Geometry check sheet. Reference: the model listing, model coordinates, mm. Round coordinates to 2 decimals unless told otherwise and drop trailing zeros. Write each loop counter-clockwise with the first axis right and the second up, starting at its lowest first coordinate (ties: lowest second). Pieces come first, ordered by that corner, then holes. Notation, with made-up numbers: (16, 57.5) - (43, 57.5) arc R14 ccw to (43, 77.5) - close; hole circle Ø8 at (60, -16.5). An arc over 180 degrees is marked (long way). Return JSON: item names as keys, results as strings.
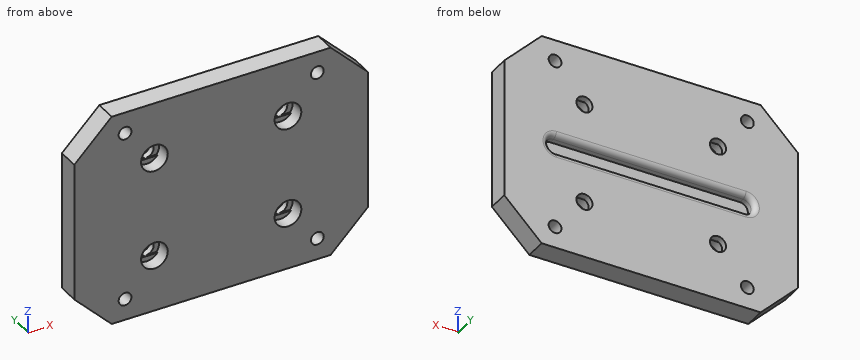
```python
from build123d import *

# Parameters (mm, degrees)
SKETCH2_W           = 55
SKETCH2_H           = 40
SKETCH2_R           = 1.2
BOSS_EXTRUDE1_DEPTH = 4
CHAMFER1_SIZE       = 7
SKETCH3_R           = 1.5
CUT_EXTRUDE1_DEPTH  = 35.062442661
FILLET1_R           = 1
CUT_EXTRUDE2_START  = 0.5
SKETCH4_R           = 2.5
CUT_EXTRUDE2_DEPTH  = 35.562442661
CUT_EXTRUDE6_START  = 0.3
CUT_EXTRUDE6_DEPTH  = 0.3


with BuildPart() as part:
    # Sketch2 → Boss-Extrude1 (new body)
    with BuildSketch(Plane(origin=(0, 0, 0), x_dir=(1, 0, 0), z_dir=(0, 1, 0))):
        Rectangle(SKETCH2_W, SKETCH2_H)
        with Locations(Location((-18, -16, 0), (0, 0, 270))):
            Circle(SKETCH2_R, mode=Mode.SUBTRACT)
        with Locations(Location((18, -16, 0), (0, 0, 270))):
            Circle(SKETCH2_R, mode=Mode.SUBTRACT)
        with Locations(Location((-18, 16, 0), (0, 0, 270))):
            Circle(SKETCH2_R, mode=Mode.SUBTRACT)
        with Locations(Location((18, 16, 0), (0, 0, 270))):
            Circle(SKETCH2_R, mode=Mode.SUBTRACT)
    extrude(amount=-BOSS_EXTRUDE1_DEPTH)

    # Chamfer1
    chamfer1_edges = [part.edges().sort_by_distance(p)[0] for p in [
        (27.5, -2, 20),
        (-27.5, -2, 20),
        (-27.5, -2, -20),
        (27.5, -2, -20),
    ]]
    chamfer(chamfer1_edges, length=CHAMFER1_SIZE)

    # Sketch3 → Cut-Extrude1 (cut, through all)
    with BuildSketch(Plane(origin=(0, -2, 0), x_dir=(1, 0, 0), z_dir=(0, 1, 0))):
        with Locations(Location((12.5, 9.4, 0), (0, 0, 270))):
            Circle(SKETCH3_R)
        with Locations(Location((-12.5, 9.4, 0), (0, 0, 270))):
            Circle(SKETCH3_R)
        with Locations(Location((-12.5, -9.4, 0), (0, 0, 270))):
            Circle(SKETCH3_R)
        with Locations(Location((12.5, -9.4, 0), (0, 0, 270))):
            Circle(SKETCH3_R)
        with BuildLine():
            Line((17.75, 1.5), (-17.75, 1.5))
            ThreePointArc((-17.75, 1.5), (-19.25, 0), (-17.75, -1.5))
            Line((-17.75, -1.5), (17.75, -1.5))
            ThreePointArc((17.75, -1.5), (19.25, 0), (17.75, 1.5))
        make_face()
    extrude(amount=CUT_EXTRUDE1_DEPTH, mode=Mode.SUBTRACT)

    # Fillet1
    fillet1_edges = [part.edges().sort_by_distance(p)[0] for p in [
        (19.25, 0, 0),
        (0, 0, -1.5),
        (-19.25, 0, 0),
        (0, 0, 1.5),
    ]]
    fillet(fillet1_edges, radius=FILLET1_R)

    # Sketch4 → Cut-Extrude2 (cut, through all)
    with BuildSketch(Plane(origin=(0, -2, 0), x_dir=(1, 0, 0), z_dir=(0, 1, 0)).offset(CUT_EXTRUDE2_START)):
        with Locations(Location((-12.5, 9.4, 0), (0, 0, 270))):
            Circle(SKETCH4_R)
        with Locations(Location((12.5, 9.4, 0), (0, 0, 270))):
            Circle(SKETCH4_R)
        with Locations(Location((-12.5, -9.4, 0), (0, 0, 270))):
            Circle(SKETCH4_R)
        with Locations(Location((12.5, -9.4, 0), (0, 0, 270))):
            Circle(SKETCH4_R)
    extrude(amount=-CUT_EXTRUDE2_DEPTH, mode=Mode.SUBTRACT)

    # Sketch5 → Cut-Extrude6 (cut)
    with BuildSketch(Plane(origin=(0, -1.5, 0), x_dir=(1, 0, 0), z_dir=(0, 1, 0)).offset(CUT_EXTRUDE6_START)):
        with BuildLine():
            Line((-14.5, -10.9), (-10.5, -10.9))
            ThreePointArc((-10.5, -10.9), (-10, -9.4), (-10.5, -7.9))
            Line((-10.5, -7.9), (-14.5, -7.9))
            ThreePointArc((-14.5, -7.9), (-15, -9.4), (-14.5, -10.9))
        make_face()
        with BuildLine():
            Line((-14.5, 7.9), (-10.5, 7.9))
            ThreePointArc((-10.5, 7.9), (-10, 9.4), (-10.5, 10.9))
            Line((-10.5, 10.9), (-14.5, 10.9))
            ThreePointArc((-14.5, 10.9), (-15, 9.4), (-14.5, 7.9))
        make_face()
        with BuildLine():
            Line((10.5, -10.9), (14.5, -10.9))
            ThreePointArc((14.5, -10.9), (15, -9.4), (14.5, -7.9))
            Line((14.5, -7.9), (10.5, -7.9))
            ThreePointArc((10.5, -7.9), (10, -9.4), (10.5, -10.9))
        make_face()
        with BuildLine():
            Line((10.5, 7.9), (14.5, 7.9))
            ThreePointArc((14.5, 7.9), (15, 9.4), (14.5, 10.9))
            Line((14.5, 10.9), (10.5, 10.9))
            ThreePointArc((10.5, 10.9), (10, 9.4), (10.5, 7.9))
        make_face()
    extrude(amount=-CUT_EXTRUDE6_DEPTH, mode=Mode.SUBTRACT)


solid = part.part
```
(1) Section check A-A, the plane z = 16. Enter the section's corners in (x, y), plus the area to 3 significant figures.
Response values:
{"outline": "(-24.5, -4) - (-19.2, -4) - (-19.2, 0) - (-24.5, 0) - close; (-16.8, -4) - (16.8, -4) - (16.8, 0) - (-16.8, 0) - close; (19.2, -4) - (24.5, -4) - (24.5, 0) - (19.2, 0) - close", "area": "177 mm^2"}
(2) Section check D-D, the plane z = 9.4. Enter the section's corners in (x, y), plus the area to 3 significant figures.
Response values:
{"outline": "(-27.5, -4) - (-15, -4) - (-15, -1.2) - (-14, -1.2) - (-14, 0) - (-27.5, 0) - close; (-11, -1.2) - (-10, -1.2) - (-10, -4) - (10, -4) - (10, -1.2) - (11, -1.2) - (11, 0) - (-11, 0) - close; (14, -1.2) - (15, -1.2) - (15, -4) - (27.5, -4) - (27.5, 0) - (14, 0) - close", "area": "185 mm^2"}
(3) Material ranges on line 1 along X through (y, z) = (-3.3, 9.5); line 2 along X through (y, z) = (-0.75, 9.4); line 3 along Z through (x, y) = (-12.5, -0.9), recorded low to high. Write a range as [from, to].
Response values:
{"line 1": "x = [-27.5, -15], [-10, 10], [15, 27.5]", "line 2": "x = [-27.5, -14], [-11, 11], [14, 27.5]", "line 3": "z = [-20, -10.9], [-7.9, -1.51], [1.51, 7.9], [10.9, 20]"}
(4) Section check C-C, the plane y = -2.55. Give the number of separate pieces and of enclosed holes in the cut face, plus the area to 3 significant figures.
Response values:
{"separate pieces": "1", "enclosed holes": "8", "area": "2,010 mm^2"}
(5) Section check B-B, the plane x = -7. Enter the section's corners in (y, z).
Response values:
{"outline": "(-4, -20) - (0, -20) - (0, -2.5) arc R1 ccw to (-1, -1.5) - (-2, -1.5) - (-2, 1.5) - (-1, 1.5) arc R1 ccw to (0, 2.5) - (0, 20) - (-4, 20) - close"}
(6) Gauge pin test, flat ends, axial feed: pin 1 (3 mm diameter, centred on x = 12, z = 9, fed in from -Y); pin 2 (1.4 mm diameter, centred on x = -18, z = -16, fed in from -Y); pin 3 (0.8 mm diameter, centred on x = 14, z = -10, fed in from -Y). Record the tip position at first contact, or that the pin passes through.
Response values:
{"pin 1": "stops at y = -1.5", "pin 2": "passes through", "pin 3": "stops at y = -1.2"}
